from build123d import *

# Parameters (mm, degrees)
BOSS_EXTRU_1_DEPTH      = 2
ESQUISSE2_W             = 230
ESQUISSE2_H             = 10
BOSS_EXTRU_2_DEPTH      = 2
CONG_1_R                = 1
ESQUISSE3_R             = 4.2
ENL_V_MAT_EXTRU_1_DEPTH = 285.197114693
ESQUISSE5_R             = 2.1
ENL_V_MAT_EXTRU_2_DEPTH = 385.317577012
ESQUISSE6_R             = 2.1
ENL_V_MAT_EXTRU_3_DEPTH = 285.197114693
CONG_2_R                = 10


with BuildPart() as part:
    # Esquisse1 → Boss.-Extru.1 (new body)
    with BuildSketch(Plane.XY):
        Polygon((140, -60), (-70, 150), (-140, 150), (-240, 150), (-140, -23.205080757), (-140, -150), (90, -150), (140, -100), align=None)
    extrude(amount=BOSS_EXTRU_1_DEPTH)

    # Esquisse2 → Boss.-Extru.2 (add)
    with BuildSketch(Plane.XZ.offset(150)):
        with Locations((-25, 5)):
            Rectangle(ESQUISSE2_W, ESQUISSE2_H)
    extrude(amount=BOSS_EXTRU_2_DEPTH)

    # Congé1
    cong_1_edges = [part.edges().sort_by_distance(p)[0] for p in [
        (-25, -152, 0),
        (-25, -150, 2),
    ]]
    fillet(cong_1_edges, radius=CONG_1_R)

    # Esquisse3 → Enlèv. mat.-Extru.1 (cut, through all)
    with BuildSketch(Plane.XY.offset(2)):
        with Locations((-133.564064606, 132.10753113)):
            Circle(ESQUISSE3_R)
        with Locations((5, -107.89246887)):
            Circle(ESQUISSE3_R)
        with Locations((115, -92.89246887)):
            Circle(ESQUISSE3_R)
    extrude(amount=-ENL_V_MAT_EXTRU_1_DEPTH, mode=Mode.SUBTRACT)

    # Esquisse5 → Enlèv. mat.-Extru.2 (cut, through all)
    with BuildSketch(Plane(origin=(0, -150, 0), x_dir=(1, 0, 0), z_dir=(0, 1, 0))):
        with Locations(Location((15, -6, 0), (0, 0, 270))):
            Circle(ESQUISSE5_R)
        with Locations(Location((-120, -6, 0), (0, 0, 270))):
            Circle(ESQUISSE5_R)
    extrude(amount=-ENL_V_MAT_EXTRU_2_DEPTH, mode=Mode.SUBTRACT)

    # Esquisse6 → Enlèv. mat.-Extru.3 (cut, through all)
    with BuildSketch(Plane.XY.offset(2)):
        with Locations((123.388347648, -50.45941546)):
            Circle(ESQUISSE6_R)
        with Locations((-60.45941546, 133.388347648)):
            Circle(ESQUISSE6_R)
    extrude(amount=-ENL_V_MAT_EXTRU_3_DEPTH, mode=Mode.SUBTRACT)

    # Congé2
    cong_2_edges = [part.edges().sort_by_distance(p)[0] for p in [
        (-140, -23.205080757, 1),
    ]]
    fillet(cong_2_edges, radius=CONG_2_R)


solid = part.part
Geometry check sheet. Reference: the model listing, model coordinates, mm. A direction names the side the tool comes from. Coordinates: 2 decimals unless noted, no trailing zeros. Write each loop counter-clockwise with the first axis right and the second up, starting at its lowest first coordinate (ties: lowest second). Pieces come first, ordered by that corner, then holes. Notation, with made-up numbers: (-34.75, 88) -> (-23.75, 88) arc R24 ccw to (-23.75, 99) -> close; hole circle Ø1 at (19.5, 43.5). An arc over 180 degrees is marked (long way). One line per question, with ' | ' between items.
1. Thickness scan on probe 1 along X at (y, z) = (-150.6, 6); probe 2 along X at (y, z) = (133, 1.5); probe 3 along Z at (x, y) = (-57.5, 78). Record the ranges inside material, lowest first. Write a range as from..to.
Answers:
probe 1: x = -140..-122.1, -117.9..12.9, 17.1..90 | probe 2: x = -230.19..-137.67, -129.46..-62.52, -58.4..-53 | probe 3: z = 0..2
2. Cross-section at D-D on y = -122. Record the cut outline in (x, z).
Answers:
outline: (-140, 0) -> (118, 0) -> (118, 2) -> (-140, 2) -> close
3. Cross-section at C-C on x = -37.5. Record the cut outline in (y, z), and give its area (3 significant figures).
Answers:
outline: (-152, 1) arc R1 ccw to (-151, 0) -> (117.5, 0) -> (117.5, 2) -> (-149, 2) arc R1 cw to (-150, 3) -> (-150, 10) -> (-152, 10) -> close | area: 555 mm²
4. Cross-section at A-A on x = 115. Record the cut outline in (y, z).
Answers:
outline: (-125, 0) -> (-97.09, 0) -> (-97.09, 2) -> (-125, 2) -> close; (-88.69, 0) -> (-35, 0) -> (-35, 2) -> (-88.69, 2) -> close
5. Draft check along X on faces 4 (the flat face through (-27, -152, 6)), 5 (the flat face through (115, -125, 1)), 6 (the cylindrical face through (4.09, -111.993, 1.014)), 7 (the cylindrical face through (-137.76, 132.29, 1.01)). Enter one of: +X half, -X half, draft (parallel to the pull), parting line (faces both ways), or undercut.
Answers:
face 4: draft | face 5: +X half | face 6: undercut | face 7: undercut
6. Set-up check for faces 1 (the flat face through (36, 44, 1)), 2 (the flat face through (-53, 3, 2)), 3 (the flat face through (-140, -89, 1)): record each of +Z, -Z, +X, -X, +Y, -Y from which the full face is reachable in a straight line by a thin tool's end or side.
Answers:
face 1: +Z, -Z, +X, +Y | face 2: +Z, +X, -X, +Y | face 3: +Z, -Z, -X, -Y
7. Cross-section at B-B on z = 6. Record the cut outline in (x, y), and give its area (3 significant figures).
Answers:
outline: (-140, -152) -> (-122.1, -152) -> (-122.1, -150) -> (-140, -150) -> close; (-117.9, -152) -> (12.9, -152) -> (12.9, -150) -> (-117.9, -150) -> close; (17.1, -152) -> (90, -152) -> (90, -150) -> (17.1, -150) -> close | area: 443 mm²
8. Depth check by flat-ended pin: pin 1 Ø13.5 at (x, y) = (115, -92.89) entering from +Z; pin 2 Ø2 at (y, z) = (-151, 6) entering from +X. Enter the tip coordinate at first touch or a pass-through.
Answers:
pin 1: stops at z = 2 | pin 2: stops at x = 90
